Source: CAD feature listing. Evaluate the final solid. Frame: model axes, mm. A direction names the side the tool comes from. Give positions to 0.01 mm unless a question says otherwise; leave off trailing zeros. Write each loop counter-clockwise with the first axis right and the second up, starting at its lowest first coordinate (ties: lowest second). Pieces come first, ordered by that corner, then holes. Notation, with made-up numbers: M 85,56 L 135,56 A12 ccw 135,62 Z; hole C -8,87 d4. An arc over 180 degrees is marked long. Return JSON: item names as keys, results as strings.
```python
from build123d import *

# Parameters (mm, degrees)
SKETCH1_W           = 12
SKETCH1_H           = 12
BOSS_EXTRUDE1_DEPTH = 12
SKETCH2_W           = 0.972972973
SKETCH2_H           = 11
CUT_EXTRUDE1_DEPTH  = 21.784609691
LPATTERN1_COUNT     = 7
LPATTERN1_PITCH     = 1.621621622


with BuildPart() as part:
    # Sketch1 → Boss-Extrude1 (new body)
    with BuildSketch(Plane(origin=(0, 0, 0), x_dir=(1, 0, 0), z_dir=(0, 1, 0))):
        with Locations((-6, -6)):
            Rectangle(SKETCH1_W, SKETCH1_H)
    extrude(amount=BOSS_EXTRUDE1_DEPTH)

    # Sketch2 → Cut-Extrude1 (cut, through all)
    with BuildSketch(Plane.XY.offset(12)):
        with Locations((-10.864864864, 6.5)):
            Rectangle(SKETCH2_W, SKETCH2_H)
    cut_extrude1 = extrude(amount=-CUT_EXTRUDE1_DEPTH, mode=Mode.SUBTRACT)

    # LPattern1: Cut-Extrude1 ×7
    with Locations(*[(i * LPATTERN1_PITCH, 0, 0) for i in range(1, LPATTERN1_COUNT)]):
        add(cut_extrude1, mode=Mode.SUBTRACT)


solid = part.part
```
1) Draft query along X for faces 1 (the face through (-6, 0, 6)), 2 (the face through (-1.622, 6, 6)). Return one class per face: released by +X, released by -X, zero draft, split by the parting line, or undercut.
Numbers:
{"face 1": "zero draft", "face 2": "undercut"}
2) Contact query for a flat-ended pin moving along its axis: pin 1 Ø0.5 at (x, z) = (-7.5, 6) entering from +Y. Output: stop coordinate, or through.
Numbers:
{"pin 1": "stops at y = 1"}
3) Cut plane A-A, the plane y = 1.5. Give the number of separate pieces and of enclosed holes in the cut face, then the cut area to 3 significant figures.
Numbers:
{"separate pieces": "8", "enclosed holes": "0", "area": "62.3 mm²"}
4) Cut plane C-C, the plane x = -6. Return the cut outline in (y, z), then the cut area to 3 significant figures.
Numbers:
{"outline": "M 0,0 L 1,0 L 1,12 L 0,12 Z", "area": "12.0 mm²"}
5) Line query: line 1 (Y direction, x = -7.75, z = 6.5). Output: solid intervals per line, ascending. Write a range as [from, to].
Numbers:
{"line 1": "y = [0, 1]"}
6) Set-up query: faces 3 (the face through (-6, 1, 6)), 4 (the face through (-10, 6, 0)). Return all of +Z, -Z, +X, -X, +Y, -Y with unobstructed straight access to the full face (end or side cutting, diameter ignored); none if empty.
Numbers:
{"face 3": "+Z, -Z, +Y", "face 4": "-Z, +X, -X, +Y, -Y"}
